CAD build for the part. Positions are in the model's coordinates, mm. Face numbers are marked on the shaded views. A direction names the side the tool comes from. Coordinates: 2 decimals unless noted, no trailing zeros. Loops run counter-clockwise (first coordinate to the right, second up) from the corner with the lowest first, then second, coordinate; pieces in that order, holes last. Notation, with made-up numbers: (66.5, 34) - (122.5, 34) arc R14 cw to (122.5, 48) - close; hole circle Ø1 at (-33.75, 52). An arc over 180 degrees is marked (long way). Put each result on its own line as item: value.
```python
from build123d import *

# Parameters (mm, degrees)
SKETCH1_R                = 7
BOSS_EXTRUDE1_DEPTH      = 20
BOSS_EXTRUDE2_DEPTH      = 10
BOSS_EXTRUDE2_DEPTH_BACK = 40
CUT_EXTRUDE1_START       = -72
CUT_EXTRUDE1_DEPTH       = 72
BOSS_EXTRUDE5_START      = -40
BOSS_EXTRUDE5_DEPTH      = 40
CUT_EXTRUDE3_START       = -10
CUT_EXTRUDE3_DEPTH       = 10
CUT_EXTRUDE5_REACH       = 91.582
CUT_EXTRUDE5_END_RADIUS  = 40
SKETCH11_W               = 30
SKETCH11_H               = 20
SKETCH12_R               = 7.5
CUT_EXTRUDE6_DEPTH       = 70


with BuildPart() as part:
    # Sketch1 → Boss-Extrude1 (new body)
    with BuildSketch(Plane(origin=(0, 0, 0), x_dir=(1, 0, 0), z_dir=(0, 1, 0))):
        with BuildLine():
            Line((-55, 15), (55, 15))
            ThreePointArc((55, 15), (70, 0), (55, -15))
            Line((55, -15), (-55, -15))
            ThreePointArc((-55, -15), (-70, 0), (-55, 15))
        make_face()
        with Locations(Location((-55, 0, 0), (0, 0, 270))):
            Circle(SKETCH1_R, mode=Mode.SUBTRACT)
        with Locations(Location((55, 0, 0), (0, 0, 270))):
            Circle(SKETCH1_R, mode=Mode.SUBTRACT)
    extrude(amount=-BOSS_EXTRUDE1_DEPTH)

    # Sketch2 → Boss-Extrude2 (add, two sides: drawn at the far end of the back side and taken through both)
    with BuildSketch(Plane.XY.offset(15).offset(-BOSS_EXTRUDE2_DEPTH_BACK)):
        with BuildLine():
            Line((-40, -20), (-35, -20))
            Line((-35, -20), (-35, -15))
            Line((-35, -15), (-29.580398915, -15))
            ThreePointArc((-29.580398915, -15), (0, 10), (29.580398915, -15))
            Line((29.580398915, -15), (35, -15))
            Line((35, -15), (35, -20))
            Line((35, -20), (40, -20))
            ThreePointArc((40, -20), (0, 20), (-40, -20))
        make_face()
    extrude(amount=BOSS_EXTRUDE2_DEPTH + BOSS_EXTRUDE2_DEPTH_BACK)

    # Sketch3 → Cut-Extrude1 (cut)
    with BuildSketch(Plane.XY.offset(15).offset(CUT_EXTRUDE1_START)):
        with BuildLine():
            Line((-35, -20), (-35, -15))
            Line((-35, -15), (-29.580398915, -15))
            ThreePointArc((-29.580398915, -15), (0, 10), (29.580398915, -15))
            Line((29.580398915, -15), (35, -15))
            Line((35, -15), (35, -20))
            Line((35, -20), (-35, -20))
        make_face()
    extrude(amount=CUT_EXTRUDE1_DEPTH, mode=Mode.SUBTRACT)

    # Sketch7 → Boss-Extrude5 (add)
    with BuildSketch(Plane.XY.offset(25).offset(BOSS_EXTRUDE5_START)):
        with BuildLine():
            Line((-20, 30), (20, 30))
            Line((20, 30), (20, 14.641016151))
            ThreePointArc((20, 14.641016151), (0, 20), (-20, 14.641016151))
            Line((-20, 14.641016151), (-20, 30))
        make_face()
    extrude(amount=BOSS_EXTRUDE5_DEPTH)

    # Sketch10 → Cut-Extrude3 (cut)
    with BuildSketch(Plane.XY.offset(25).offset(CUT_EXTRUDE3_START)):
        with BuildLine():
            Line((-20, 14.641016151), (-20, 30))
            Line((-20, 30), (20, 30))
            Line((20, 30), (20, 14.641016151))
            ThreePointArc((20, 14.641016151), (0, 20), (-20, 14.641016151))
        make_face()
    extrude(amount=CUT_EXTRUDE3_DEPTH, mode=Mode.SUBTRACT)

    # Cut-Extrude5: up to this cylinder (the profile starts outside it)
    cut_extrude5_end = Plane(origin=(0, -20, 0), z_dir=(0, 0, 1)) * Cylinder(CUT_EXTRUDE5_END_RADIUS, 264.164, mode=Mode.PRIVATE)
    # Sketch11 → Cut-Extrude5 (cut, up to the surface)
    with BuildSketch(Plane(origin=(0, 30, 0), x_dir=(1, 0, 0), z_dir=(0, 1, 0)), mode=Mode.PRIVATE) as cut_extrude5_sk1:
        Rectangle(SKETCH11_W, SKETCH11_H)
    cut_extrude5_tool1 = extrude(cut_extrude5_sk1.sketch, amount=-CUT_EXTRUDE5_REACH, mode=Mode.PRIVATE) - cut_extrude5_end
    add(cut_extrude5_tool1.solids().sort_by_distance((0, 30, 0))[0], mode=Mode.SUBTRACT)

    # Sketch12 → Cut-Extrude6 (cut)
    with BuildSketch(Plane(origin=(0, 30, 0), x_dir=(1, 0, 0), z_dir=(0, 1, 0))):
        with Locations(Location((0, 0, 0), (0, 0, 270))):
            Circle(SKETCH12_R)
    extrude(amount=-CUT_EXTRUDE6_DEPTH, mode=Mode.SUBTRACT)


solid = part.part
```
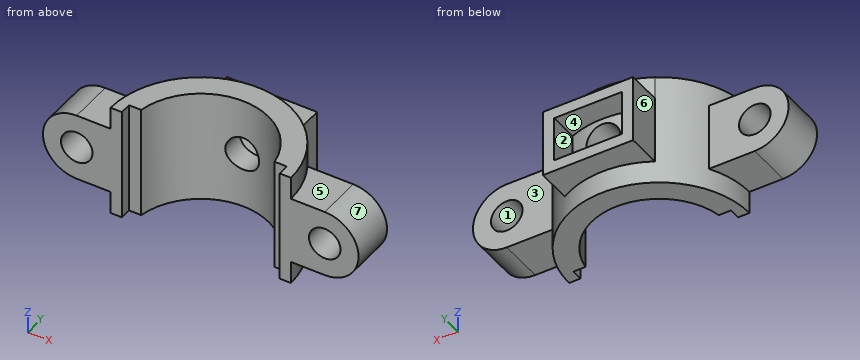
Q1. Slice it at D-D, the plane y = 25.5. Give the cut face in (x, z).
Determined:
outline: (-20, -15) - (20, -15) - (20, 15) - (-20, 15) - close; hole (-15, -10) - (15, -10) - (15, 10) - (-15, 10) - close
Q2. Slice it at A-A, the plane y = -3. Give the cut face in (x, z), then the cut area to 3 significant figures.
Determined:
outline: (-55, -15) - (-36.21, -15) - (-36.21, -25) - (-24.72, -25) - (-24.72, 25) - (-36.21, 25) - (-36.21, 15) - (-55, 15) arc R15 ccw to start; (24.72, -25) - (36.21, -25) - (36.21, -15) - (55, -15) arc R15 ccw to (55, 15) - (36.21, 15) - (36.21, 25) - (24.72, 25) - close; hole circle Ø14 at (-55, 0); hole circle Ø14 at (55, 0)
area: 2,680 mm2
Q3. Wall check: L1, parallel to Z at x = 2.5, y = 20; L2, parallel to X at y = -7.5, z = 0; L3, parallel to X at y = -9, z = 0. Give the ranges that are in metal, low to high. Write a range as from..to.
Determined:
L1: -15..-10, 10..15
L2: -70..-62, -48..-27.27, 27.27..48, 62..70
L3: -70..-62, -48..-27.91, 27.91..48, 62..70
Q4. Tool access for the marked faces 1, 2 and 3: list every direction of +Z, -Z, +X, -X, +Y, -Y with a clear straight run to the whole face (end or side of a thin tool).
Determined:
face 1: +Y, -Y
face 2: +Y
face 3: +Z, -Z, +X, +Y
Q5. Mould opens along X. For the marked faces 4, 5, 6 and 7 say: +X half, -X half, draft (parallel to the pull), parting line (faces both ways), or undercut.
Determined:
face 4: undercut
face 5: draft
face 6: -X half
face 7: +X half
Q6. Slice it at B-B, the plane x = 0. Give the cut face in (y, z).
Determined:
outline: (10, -25) - (20, -25) - (20, -15) - (30, -15) - (30, -10) - (20, -10) - (20, -7.5) - (10, -7.5) - close; (10, 7.5) - (20, 7.5) - (20, 10) - (30, 10) - (30, 15) - (20, 15) - (20, 25) - (10, 25) - close
Q7. Slice it at C-C, the plane z = -1. State how many separate pieces and enclosed holes the cut face has, then the cut area to 3 significant figures.
Determined:
separate pieces: 4
enclosed holes: 0
area: 1,750 mm2
Q8. Pin check, flat tips, straight feed: pin 1 Ø1.5 at (x, z) = (-8.5, -0.5) entering from -Y; pin 2 Ø10 at (y, z) = (12.5, -4) entering from -X; pin 3 Ø4 at (x, y) = (-0.5, 25) entering from -Z. Stop position of each tip, or through.
Determined:
pin 1: y = 8.54
pin 2: x = -29.05
pin 3: z = -15
